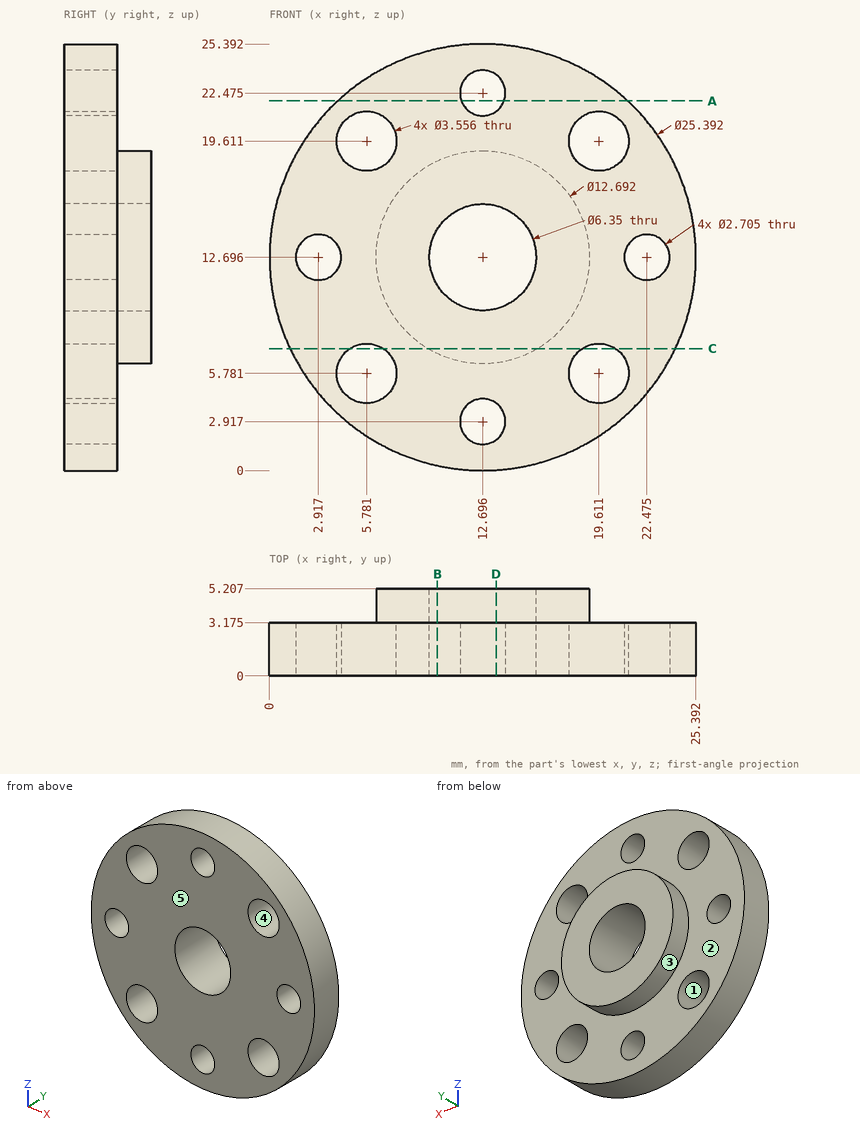
For this review, use the dimensioned drawing (mm, ordinates from the lowest corner) and the shaded views. A direction names the side the tool comes from. Coordinates: 2 decimals unless noted, no trailing zeros. Loops run counter-clockwise (first coordinate to the right, second up) from the corner with the lowest first, then second, coordinate; pieces in that order, holes last.
1. Add section C-C, the plane z = 7.25. Give the boundary of the cut face in (x, y) (1 decimal).
2. For line 1 (Z direction, x = 18.75, y = 2.85) (1 decimal); line 2 (Y direction, x = 11.5, z = 1.5) (1 decimal); line 3 (Z direction, x = 10, y = 2.05) (1 decimal), list the stretches that pass through material, from the lowest coordinate up.
3. Mouldability with a two-part tool opening along X and no side actions: class the marked faces 3, 4 and 5 as +X half, -X half, draft (parallel to the pull), parting line (faces both ways), or undercut.
4. Insertion check: P1, Ø12, axis at x = 9.5, z = 14, coming from the -Y side; P2, Ø3, axis at x = 19.61, z = 5.78, coming from the +Y side; P3, Ø1.5, axis at x = 11, z = 20.5, coming from the +Y side (3 decimals); P4, Ø1, axis at y = 2.5, z = 21.5, coming from the +X side. Each pin has a flat end and moves straight along its axis. Give the tip position at first contact, or say it passes through.
5. Add section A-A, the plane z = 22. Give the boundary of the cut face in (x, y) (1 decimal), then the cut area to 3 significant figures.
6. Add section B-B, the plane x = 10. Give the boundary of the cut face in (y, z) (1 decimal).
7. For the marked faces 1 and 2, list the 3-axis set-ups (+Z, -Z, +X, -X, +Y, -Y) from which the entire face can be reached by the end or side of a thin tool; tool diameter is ignored.
8. Add section D-D, the plane x = 13.5. Give the boundary of the cut face in (y, z) (1 decimal).
Result:
1. outline: (1.2, 0) - (4.8, 0) - (4.8, 3.2) - (1.2, 3.2) - close; (6.8, 0) - (18.6, 0) - (18.6, 3.2) - (16, 3.2) - (16, 5.2) - (9.4, 5.2) - (9.4, 3.2) - (6.8, 3.2) - close; (20.6, 0) - (24.2, 0) - (24.2, 3.2) - (20.6, 3.2) - close
2. line 1: z = 1.5 to 4.2, 7.3 to 18.1, 21.2 to 23.9
2. line 2: y = 0 to 3.2
2. line 3: z = 0.3 to 11, 14.4 to 25.1
3. face 3: parting line
3. face 4: undercut
3. face 5: draft
4. P1: stops at y = 0
4. P2: passes through
4. P3: stops at y = 3.175
4. P4: stops at x = 22.3
5. outline: (4.1, 0) - (11.4, 0) - (11.4, 3.2) - (4.1, 3.2) - close; (14, 0) - (21.3, 0) - (21.3, 3.2) - (14, 3.2) - close
5. area: 46.8 mm2
6. outline: (0, 0.3) - (3.2, 0.3) - (3.2, 7) - (5.2, 7) - (5.2, 11) - (0, 11) - close; (0, 14.4) - (5.2, 14.4) - (5.2, 18.4) - (3.2, 18.4) - (3.2, 25.1) - (0, 25.1) - close
7. face 1: +Y, -Y
7. face 2: +Y
8. outline: (0, 0) - (3.2, 0) - (3.2, 1.8) - (0, 1.8) - close; (0, 4) - (3.2, 4) - (3.2, 6.4) - (5.2, 6.4) - (5.2, 9.6) - (0, 9.6) - close; (0, 15.8) - (5.2, 15.8) - (5.2, 19) - (3.2, 19) - (3.2, 21.4) - (0, 21.4) - close; (0, 23.6) - (3.2, 23.6) - (3.2, 25.4) - (0, 25.4) - close
